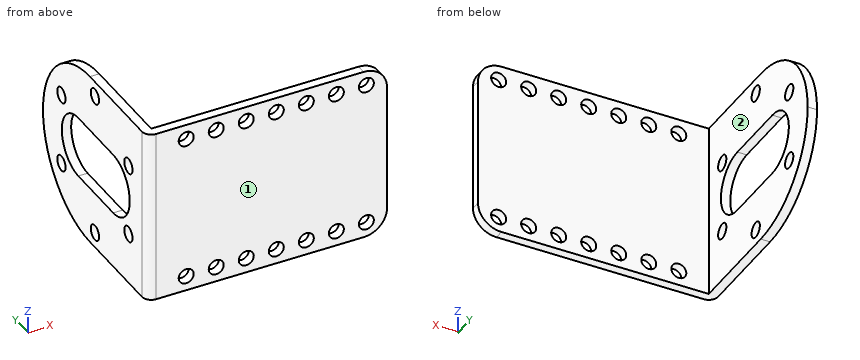
from build123d import *

# Parameters (mm, degrees)
SKETCH1_W           = 51.2
SKETCH1_H           = 37.6
SKETCH1_R           = 1.6
BOSS_EXTRUDE1_DEPTH = 2
FILLET2_R           = 5
SKETCH2_W           = 2
SKETCH2_H           = 37.6
BOSS_EXTRUDE2_DEPTH = 39.6
CUT_EXTRUDE1_REACH  = 70.596
SKETCH3_R           = 1.65
FILLET3_R           = 18.8
FILLET4_R           = 2


with BuildPart() as part:
    # Sketch1 → Boss-Extrude1 (new body)
    with BuildSketch(Plane(origin=(0, 0, 0), x_dir=(1, 0, 0), z_dir=(0, 1, 0))):
        Rectangle(SKETCH1_W, SKETCH1_H)
        with Locations(Location((-17.2, 15.6, 0), (0, 0, 270))):
            Circle(SKETCH1_R, mode=Mode.SUBTRACT)
        with Locations(Location((-10.8, 15.6, 0), (0, 0, 270))):
            Circle(SKETCH1_R, mode=Mode.SUBTRACT)
        with Locations(Location((-4.4, 15.6, 0), (0, 0, 270))):
            Circle(SKETCH1_R, mode=Mode.SUBTRACT)
        with Locations(Location((2, 15.6, 0), (0, 0, 270))):
            Circle(SKETCH1_R, mode=Mode.SUBTRACT)
        with Locations(Location((8.4, 15.6, 0), (0, 0, 270))):
            Circle(SKETCH1_R, mode=Mode.SUBTRACT)
        with Locations(Location((14.8, 15.6, 0), (0, 0, 270))):
            Circle(SKETCH1_R, mode=Mode.SUBTRACT)
        with Locations(Location((21.2, 15.6, 0), (0, 0, 270))):
            Circle(SKETCH1_R, mode=Mode.SUBTRACT)
        with Locations(Location((21.2, -15.6, 0), (0, 0, 90))):
            Circle(SKETCH1_R, mode=Mode.SUBTRACT)
        with Locations(Location((14.8, -15.6, 0), (0, 0, 90))):
            Circle(SKETCH1_R, mode=Mode.SUBTRACT)
        with Locations(Location((8.4, -15.6, 0), (0, 0, 90))):
            Circle(SKETCH1_R, mode=Mode.SUBTRACT)
        with Locations(Location((2, -15.6, 0), (0, 0, 90))):
            Circle(SKETCH1_R, mode=Mode.SUBTRACT)
        with Locations(Location((-4.4, -15.6, 0), (0, 0, 90))):
            Circle(SKETCH1_R, mode=Mode.SUBTRACT)
        with Locations(Location((-10.8, -15.6, 0), (0, 0, 90))):
            Circle(SKETCH1_R, mode=Mode.SUBTRACT)
        with Locations(Location((-17.2, -15.6, 0), (0, 0, 90))):
            Circle(SKETCH1_R, mode=Mode.SUBTRACT)
    extrude(amount=BOSS_EXTRUDE1_DEPTH)

    # Fillet2
    fillet2_edges = [part.edges().sort_by_distance(p)[0] for p in [
        (25.6, 1, 18.8),
        (25.6, 1, -18.8),
    ]]
    fillet(fillet2_edges, radius=FILLET2_R)

    # Sketch2 → Boss-Extrude2 (add)
    with BuildSketch(Plane(origin=(0, 2, 0), x_dir=(1, 0, 0), z_dir=(0, 1, 0))):
        with Locations((-24.6, 0)):
            Rectangle(SKETCH2_W, SKETCH2_H)
    extrude(amount=BOSS_EXTRUDE2_DEPTH)

    # Sketch3 → Cut-Extrude1 (cut, up to next)
    with BuildSketch(Plane.ZY.offset(25.6), mode=Mode.PRIVATE) as cut_extrude1_sk1:
        with Locations((7.75, 34.223393759)):
            Circle(SKETCH3_R)
    cut_extrude1_tool1 = extrude(cut_extrude1_sk1.sketch, amount=-CUT_EXTRUDE1_REACH, mode=Mode.PRIVATE) & part.part
    # Sketch3 → Cut-Extrude1 (cut, up to next)
    with BuildSketch(Plane.ZY.offset(25.6), mode=Mode.PRIVATE) as cut_extrude1_sk2:
        with Locations((15.5, 20.8)):
            Circle(SKETCH3_R)
    cut_extrude1_tool2 = extrude(cut_extrude1_sk2.sketch, amount=-CUT_EXTRUDE1_REACH, mode=Mode.PRIVATE) & part.part
    # Sketch3 → Cut-Extrude1 (cut, up to next)
    with BuildSketch(Plane.ZY.offset(25.6), mode=Mode.PRIVATE) as cut_extrude1_sk3:
        with Locations((7.75, 7.376606241)):
            Circle(SKETCH3_R)
    cut_extrude1_tool3 = extrude(cut_extrude1_sk3.sketch, amount=-CUT_EXTRUDE1_REACH, mode=Mode.PRIVATE) & part.part
    # Sketch3 → Cut-Extrude1 (cut, up to next)
    with BuildSketch(Plane.ZY.offset(25.6), mode=Mode.PRIVATE) as cut_extrude1_sk4:
        with Locations((-7.75, 7.376606241)):
            Circle(SKETCH3_R)
    cut_extrude1_tool4 = extrude(cut_extrude1_sk4.sketch, amount=-CUT_EXTRUDE1_REACH, mode=Mode.PRIVATE) & part.part
    # Sketch3 → Cut-Extrude1 (cut, up to next)
    with BuildSketch(Plane.ZY.offset(25.6), mode=Mode.PRIVATE) as cut_extrude1_sk5:
        with Locations((-15.5, 20.8)):
            Circle(SKETCH3_R)
    cut_extrude1_tool5 = extrude(cut_extrude1_sk5.sketch, amount=-CUT_EXTRUDE1_REACH, mode=Mode.PRIVATE) & part.part
    # Sketch3 → Cut-Extrude1 (cut, up to next)
    with BuildSketch(Plane.ZY.offset(25.6), mode=Mode.PRIVATE) as cut_extrude1_sk6:
        with Locations((-7.75, 34.223393759)):
            Circle(SKETCH3_R)
    cut_extrude1_tool6 = extrude(cut_extrude1_sk6.sketch, amount=-CUT_EXTRUDE1_REACH, mode=Mode.PRIVATE) & part.part
    # Sketch3 → Cut-Extrude1 (cut, up to next)
    with BuildSketch(Plane.ZY.offset(25.6), mode=Mode.PRIVATE) as cut_extrude1_sk7:
        with BuildLine():
            Line((-6.6, 27.456121665), (-6.6, 13.456121665))
            ThreePointArc((-6.6, 13.456121665), (0, 6.856121665), (6.6, 13.456121665))
            Line((6.6, 13.456121665), (6.6, 27.456121665))
            ThreePointArc((6.6, 27.456121665), (0, 34.056121665), (-6.6, 27.456121665))
        make_face()
    cut_extrude1_tool7 = extrude(cut_extrude1_sk7.sketch, amount=-CUT_EXTRUDE1_REACH, mode=Mode.PRIVATE) & part.part
    add(cut_extrude1_tool1.solids().sort_by_distance((-25.6, 34.223394, 7.75))[0], mode=Mode.SUBTRACT)
    add(cut_extrude1_tool2.solids().sort_by_distance((-25.6, 20.8, 15.5))[0], mode=Mode.SUBTRACT)
    add(cut_extrude1_tool3.solids().sort_by_distance((-25.6, 7.376606, 7.75))[0], mode=Mode.SUBTRACT)
    add(cut_extrude1_tool4.solids().sort_by_distance((-25.6, 7.376606, -7.75))[0], mode=Mode.SUBTRACT)
    add(cut_extrude1_tool5.solids().sort_by_distance((-25.6, 20.8, -15.5))[0], mode=Mode.SUBTRACT)
    add(cut_extrude1_tool6.solids().sort_by_distance((-25.6, 34.223394, -7.75))[0], mode=Mode.SUBTRACT)
    add(cut_extrude1_tool7.solids().sort_by_distance((-25.6, 20.456122, 0))[0], mode=Mode.SUBTRACT)

    # Fillet3
    fillet3_edges = [part.edges().sort_by_distance(p)[0] for p in [
        (-24.6, 41.6, -18.8),
        (-24.6, 41.6, 18.8),
    ]]
    fillet(fillet3_edges, radius=FILLET3_R - 0.0001)  # a hair under: the kernel refuses the full size

    # Fillet4
    fillet4_edges = [part.edges().sort_by_distance(p)[0] for p in [
        (-25.6, 0, 0),
    ]]
    fillet(fillet4_edges, radius=FILLET4_R)


solid = part.part
Input: part model. Units: mm. Frame: model coordinates. Face numbers are marked on the shaded views. A direction names the side the tool comes from. Give positions to 0.01 mm unless a question says otherwise; leave off trailing zeros. Order: outer loops, then holes, each group sorted by start corner. A loop starts at its lowest first (then second) coordinate and runs counter-clockwise, first axis right, second up. Notation, with made-up numbers: (-9, 11) -> (-1, 11) arc R19 ccw to (-1, 16) -> close; hole circle Ø9 at (-25, -2). An arc over 180 degrees is marked (long way). Use one line per item in the form item = value.
1) Section B-B, the plane z = -1. Return loops of the section in (x, y), and give its area (3 significant figures).
Response values:
outline = (-25.6, 2) arc R2 ccw to (-23.6, 0) -> (25.6, 0) -> (25.6, 2) -> (-23.6, 2) -> (-23.6, 6.93) -> (-25.6, 6.93) -> close; (-25.6, 33.98) -> (-23.6, 33.98) -> (-23.6, 41.57) -> (-25.6, 41.57) -> close
area = 127 mm^2
2) Section A-A, the plane y = 17. Return loops of the section in (x, z), and give its area (3 significant figures).
Response values:
outline = (-25.6, -18.8) -> (-23.6, -18.8) -> (-23.6, -6.6) -> (-25.6, -6.6) -> close; (-25.6, 6.6) -> (-23.6, 6.6) -> (-23.6, 18.8) -> (-25.6, 18.8) -> close
area = 48.8 mm^2
3) Line query: probe 1 along Y at (x, z) = (-24.7, -7.75); probe 2 along X at (y, z) = (27, 16); probe 3 along Y at (x, z) = (-21, 16). Output: solid intervals per line, ascending.
Response values:
probe_1 = 0.33 to 5.73, 9.03 to 32.57, 35.87 to 39.93
probe_2 = -25.6 to -23.6
probe_3 = 0 to 2
4) Reachability of the marked faces 1 and 2 from +Z, -Z, +X, -X, +Y, -Y: full face, straight path, thin tool, end or side. Return the list, or none.
Response values:
face_1 = +Z, -Z, +X, -X, -Y
face_2 = +Z, -Z, +X, +Y
5) Section D-D, the plane x = -22. Return loops of the section in (y, z), and give its area (3 significant figures).
Response values:
outline = (0, -18.8) -> (2, -18.8) -> (2, 18.8) -> (0, 18.8) -> close
area = 75.2 mm^2
6) First-contact query: pin 1 Ø1.9 at (x, z) = (8.4, -15.6) entering from -Y; pin 2 Ø5 at (y, z) = (17.5, -14.5) entering from +X; pin 3 Ø1 at (x, z) = (15, -14) entering from +Y. Flat tips, straight axial feed; report the tip coordinate or a pass-through.
Response values:
pin_1 = through
pin_2 = -23.6
pin_3 = 2
7) Section C-C, the plane z = 7.75. Return loops of the section in (x, y), and give its area (3 significant figures).
Response values:
outline = (-25.6, 2) arc R2 ccw to (-23.6, 0) -> (25.6, 0) -> (25.6, 2) -> (-23.6, 2) -> (-23.6, 5.73) -> (-25.6, 5.73) -> close; (-25.6, 9.03) -> (-23.6, 9.03) -> (-23.6, 32.57) -> (-25.6, 32.57) -> close; (-25.6, 35.87) -> (-23.6, 35.87) -> (-23.6, 39.93) -> (-25.6, 39.93) -> close
area = 164 mm^2
